Source: CAD feature listing. Evaluate the final solid. Frame: model axes, mm. Face numbers are marked on the shaded views. A direction names the side the tool comes from. Round coordinates to 2 decimals unless told otherwise and drop trailing zeros. Order: outer loops, then holes, each group sorted by start corner. A loop starts at its lowest first (then second) coordinate and runs counter-clockwise, first axis right, second up.
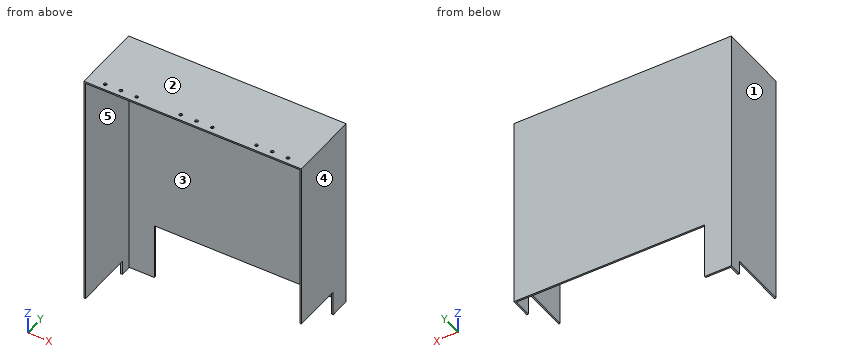
```python
from build123d import *

# Parameters (mm, degrees)
BOSS_EXTRUDE1_DEPTH = 508
SKETCH2_W           = 438.15
SKETCH2_H           = 142.875
BOSS_EXTRUDE2_DEPTH = 3.175
SKETCH4_W           = 384.175
SKETCH4_H           = 114.3
CUT_EXTRUDE1_DEPTH  = 686.895537327
CUT_EXTRUDE2_REACH  = 687.896
SKETCH5_W           = 50.8
SKETCH5_H           = 101.6
CUT_EXTRUDE3_REACH  = 687.896
SKETCH6_W           = 28.575
SKETCH6_H           = 117.475
SKETCH7_R           = 3.175
CUT_EXTRUDE4_DEPTH  = 3.175


with BuildPart() as part:
    # Sketch1 → Boss-Extrude1 (new body)
    with BuildSketch(Plane.XY):
        Polygon((0, 0), (3.175, 0), (3.175, 139.7), (434.975, 139.7), (434.975, 0), (438.15, 0), (438.15, 142.875), (0, 142.875), align=None)
    extrude(amount=BOSS_EXTRUDE1_DEPTH)

    # Sketch2 → Boss-Extrude2 (add)
    with BuildSketch(Plane.XY.offset(508)):
        with Locations((219.075, 71.4375)):
            Rectangle(SKETCH2_W, SKETCH2_H)
    extrude(amount=-BOSS_EXTRUDE2_DEPTH)

    # Sketch4 → Cut-Extrude1 (cut, through all)
    with BuildSketch(Plane(origin=(0, 142.875, 0), x_dir=(1, 0, 0), z_dir=(0, 1, 0))):
        with Locations((246.0625, -57.15)):
            Rectangle(SKETCH4_W, SKETCH4_H)
    extrude(amount=-CUT_EXTRUDE1_DEPTH, mode=Mode.SUBTRACT)

    # Sketch5 → Cut-Extrude2 (cut, up to next)
    with BuildSketch(Plane(origin=(438.15, 0, 0), x_dir=(0, 0, -1), z_dir=(1, 0, 0)), mode=Mode.PRIVATE) as cut_extrude2_sk1:
        with Locations((-139.7, 50.8)):
            Rectangle(SKETCH5_W, SKETCH5_H)
    cut_extrude2_tool1 = extrude(cut_extrude2_sk1.sketch, amount=-CUT_EXTRUDE2_REACH, mode=Mode.PRIVATE) & part.part
    add(cut_extrude2_tool1.solids().sort_by_distance((438.15, 50.8, 139.7))[0], mode=Mode.SUBTRACT)

    # Sketch6 → Cut-Extrude3 (cut, up to next)
    with BuildSketch(Plane.ZY, mode=Mode.PRIVATE) as cut_extrude3_sk1:
        with Locations((14.2875, 58.7375)):
            Rectangle(SKETCH6_W, SKETCH6_H)
    cut_extrude3_tool1 = extrude(cut_extrude3_sk1.sketch, amount=-CUT_EXTRUDE3_REACH, mode=Mode.PRIVATE) & part.part
    add(cut_extrude3_tool1.solids().sort_by_distance((0, 58.7375, 14.2875))[0], mode=Mode.SUBTRACT)

    # Sketch7 → Cut-Extrude4 (cut)
    with BuildSketch(Plane.XY.offset(508)):
        with Locations((219.075, 12.7)):
            Circle(SKETCH7_R)
        with Locations((187.325, 12.7)):
            Circle(SKETCH7_R)
        with Locations((34.925, 12.7)):
            Circle(SKETCH7_R)
        with Locations((66.675, 12.7)):
            Circle(SKETCH7_R)
        with Locations((98.425, 12.7)):
            Circle(SKETCH7_R)
        with Locations((250.825, 12.7)):
            Circle(SKETCH7_R)
        with Locations((339.725, 12.7)):
            Circle(SKETCH7_R)
        with Locations((371.475, 12.7)):
            Circle(SKETCH7_R)
        with Locations((403.225, 12.7)):
            Circle(SKETCH7_R)
    extrude(amount=-CUT_EXTRUDE4_DEPTH, mode=Mode.SUBTRACT)


solid = part.part
```
1. Pull-direction query (X, two-part tool) for the marked faces 1, 2 and 3; classes: released by +X, released by -X, zero draft, split by the parting line, or undercut.
2. Section A-A on x = 47. Return loops of the section in (y, z) (3 decimals).
3. Access query for the marked faces 4 and 5. Directions: +Z, -Z, +X, -X, +Y, -Y. A direction counts if a zero-diameter tool reaches every point of the face in a straight line with its end or side. Return the directions, or none.
4. Section B-B on y = 73. Return loops of the section in (x, z) (3 decimals), plus the area to 3 significant figures.
5. Section C-C on x = 164. Return loops of the section in (y, z) (3 decimals), plus the area to 3 significant figures.
6. First-contact query: pin 1 (2.5 mm diameter, centred on x = 436.5, y = 50, fed in from -Z); pin 2 (10 mm diameter, centred on x = 339.725, y = 12.7, fed in from -Z) (3 decimals); pin 3 (1.6 mm diameter, centred on y = 141, z = 84.5, fed in from +X) (3 decimals). Flat tips, straight axial feed; report the tip coordinate or a pass-through.
7. Line query: line 1 along X through (y, z) = (91, 456) (3 decimals); line 2 along Z through (x, y) = (339, 8) (3 decimals); line 3 along Y through (x, z) = (151.5, 373.5) (3 decimals). Output: solid intervals per line, ascending.
Result:
1. face 1: released by -X
1. face 2: zero draft
1. face 3: undercut
2. outline: (0, 504.825) - (139.7, 504.825) - (139.7, 0) - (142.875, 0) - (142.875, 508) - (0, 508) - close
3. face 4: +Z, -Z, +X, +Y, -Y
3. face 5: -Z, -Y
4. outline: (0, 28.575) - (3.175, 28.575) - (3.175, 504.825) - (434.975, 504.825) - (434.975, 165.1) - (438.15, 165.1) - (438.15, 508) - (0, 508) - close
4. area: 3,980 mm2
5. outline: (0, 504.825) - (139.7, 504.825) - (139.7, 114.3) - (142.875, 114.3) - (142.875, 508) - (0, 508) - close
5. area: 1,690 mm2
6. pin 1: stops at z = 165.1
6. pin 2: stops at z = 504.825
6. pin 3: stops at x = 53.975
7. line 1: x = 0 to 3.175, 434.975 to 438.15
7. line 2: z = 504.825 to 508
7. line 3: y = 139.7 to 142.875
